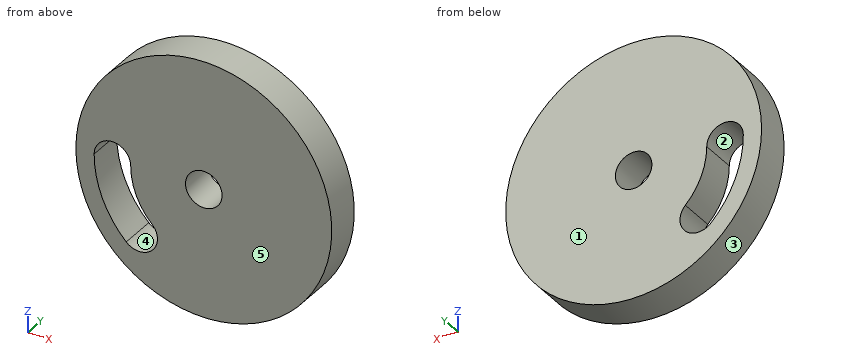
Autodesk Inventor part; units mm, degrees
ref_plane "YZ Plane" through (0, 0, 0) normal (1, 0, 0) x (0, 1, 0)
ref_plane "XZ Plane" through (0, 0, 0) normal (0, 1, 0) x (-1, 0, 0)
ref_plane "XY Plane" through (0, 0, 0) normal (0, 0, 1) x (1, 0, 0)
sketch "Sketch1" plane through (0, 0, 0) normal (0, 1, 0) x (-1, 0, 0)
  circle A0 centre (0, 0) radius 17.5
  dimension "d0" = 35
extrude "Extrusion1" add sketch "Sketch1" along normal blind 5
sketch "Sketch2" plane through (0, 5, 0) normal (0, 1, 0) x (1, 0, 0)
  arc A0 (-10.6066, 10.6066) -> (-15, 0) centre (0, 0) ccw
  line L0 (0, 0) -> (-10.6066, 10.6066) construction
  line L1 (0, 0) -> (-15, 0) construction
  arc A1 (-7.0711, 7.0711) -> (-10, 0) centre (0, 0) ccw
  arc A2 (-15, 0) -> (-10, 0) centre (-12.5, 0) ccw
  arc A3 (-7.0711, 7.0711) -> (-10.6066, 10.6066) centre (-8.8388, 8.8388) ccw
  dimension "kat" = 45
  dimension "d8" = 45
extrude "Extrusion2" cut sketch "Sketch2" against normal through all
sketch "Sketch3" plane through (0, 5, 0) normal (0, 1, 0) x (1, 0, 0)
  circle A0 centre (0, 0) radius 2.5
  dimension "d11" = 5
extrude "Extrusion3" cut sketch "Sketch3" against normal through all
Geometry: final body of the model. Coordinates: model frame, mm. Face numbers are marked on the shaded views. A direction names the side the tool comes from. Coordinates: 2 decimals unless noted, no trailing zeros. Order: outer loops, then holes, each group sorted by start corner. A loop starts at its lowest first (then second) coordinate and runs counter-clockwise, first axis right, second up.
1) Ray query, probe 1 along Z at (x, y) = (0, 1.9); probe 2 along Z at (x, y) = (-13.5, 3.7); probe 3 along X at (y, z) = (0.5, -8). Return the intervals inside material, ascending.
Result sheet:
probe 1: z = -17.5 to -2.5, 2.5 to 17.5
probe 2: z = -11.14 to -6.54, 2.29 to 11.14
probe 3: x = -15.56 to -12.69, -6.48 to 15.56
2) Set-up query: the marked faces 1 and 2. Return all of +Z, -Z, +X, -X, +Y, -Y with unobstructed straight access to the full face (end or side cutting, diameter ignored); none if empty.
Result sheet:
face 1: +Z, -Z, +X, -X, +Y
face 2: +Y, -Y
3) Section B-B (y = 1.85). Return loops of the section in (x, z).
Result sheet:
outline: circle Ø35 at (0, 0); hole (-15, 0) arc R15 ccw to (-10.61, -10.61) arc R2.5 ccw to (-7.07, -7.07) arc R10 cw to (-10, 0) arc R2.5 ccw to start; hole circle Ø5 at (0, 0)
4) Section C-C (z = -3). Return loops of the section in (x, y).
Result sheet:
outline: (-17.24, 0) - (-14.7, 0) - (-14.7, 5) - (-17.24, 5) - close; (-9.54, 0) - (17.24, 0) - (17.24, 5) - (-9.54, 5) - close
5) First-contact query: P1, Ø2, axis at x = 4.5, y = 0.5, coming from the +Z side; P2, Ø4.5, axis at x = 0, z = 0, coming from the +Y side; P3, Ø1.5, axis at x = -10.5, y = 0.5, coming from the +Z side. Flat tips, straight axial feed; report the tip coordinate or a pass-through.
Result sheet:
P1: stops at z = 17.15
P2: passes through
P3: stops at z = 14.53
6) Section D-D (x = 14). Return loops of the section in (y, z), then the cut area to 3 significant figures.
Result sheet:
outline: (0, -10.5) - (5, -10.5) - (5, 10.5) - (0, 10.5) - close
area: 105 mm2
7) Section A-A (x = 0). Return loops of the section in (y, z), then the cut area to 3 significant figures.
Result sheet:
outline: (0, -17.5) - (5, -17.5) - (5, -2.5) - (0, -2.5) - close; (0, 2.5) - (5, 2.5) - (5, 17.5) - (0, 17.5) - close
area: 150 mm2
8) Draft query along Z for the marked faces 3, 4 and 5. Return one class per face: released by +Z, released by -Z, zero draft, split by the parting line, or undercut.
Result sheet:
face 3: split by the parting line
face 4: undercut
face 5: zero draft
